Autodesk Inventor part; units mm, degrees
ref_plane "YZ Plane" through (0, 0, 0) normal (1, 0, 0) x (0, 1, 0)
ref_plane "XY Plane" through (0, 0, 0) normal (0, 0, 1) x (1, 0, 0)
sketch "Sketch1" plane through (0, 0, 0) normal (0, 0, 1) x (1, 0, 0)
  line L0 (0.9, 49.1) -> (0.9, 28.9)
  arc A0 (0.9, 49.1) -> (-0.9, 49.1) centre (0, 49.1) ccw
  line L1 (-0.9, 28.9) -> (-0.9, 49.1)
  arc A1 (-0.9, 28.9) -> (0.9, 28.9) centre (0, 28.9) ccw
  line L2 (0.9, 13.1) -> (0.9, -13.1)
  arc A2 (0.9, 13.1) -> (-0.9, 13.1) centre (0, 13.1) ccw
  line L3 (-0.9, -13.1) -> (-0.9, 13.1)
  arc A3 (-0.9, -13.1) -> (0.9, -13.1) centre (0, -13.1) ccw
  line L4 (0, 28.9) -> (0, 25.8465)
  arc A4 (0, 25.8465) -> (0.298, 23.4232) centre (10, 25.8465) ccw
  arc A5 (0.298, 18.5768) -> (0.298, 23.4232) centre (-9.4039, 21) ccw
  arc A6 (0.298, 18.5768) -> (0, 16.1535) centre (10, 16.1535) ccw
  line L5 (0, 16.1535) -> (0, 13.1)
  point P0 (0, 0)
  dimension "d0" = 10
  dimension "d1" = 10
ref_plane "Work Plane1" through (0, 28.9, 0) normal (0, 1, 0) x (-1, 0, 0)
sketch "Sketch2" plane through (0, 28.9, 0) normal (0, 1, 0) x (-1, 0, 0)
  line L0 (-0.5, 0) -> (0.5, 0)
  line L1 (0.5, 0) -> (0.5, -0.5)
  line L2 (0.5, -0.5) -> (-0.5, -0.5)
  line L3 (-0.5, -0.5) -> (-0.5, 0)
  point P0 (0, 0)
  point P1 (0, 0)
  dimension "d2" = 1
  dimension "d3" = 0.5
sweep "Sweep1" add profiles "Sketch2" path "Sketch1" path curves L4 A4 A5 A6 L5
properties part number "connector"
Verification items for the finished model (mm, model axes). Give positions to 0.01 mm unless a question says otherwise; leave off trailing zeros. Order: outer loops, then holes, each group sorted by start corner. A loop starts at its lowest first (then second) coordinate and runs counter-clockwise, first axis right, second up. Notation, with made-up numbers: M -22.5,-31.75 L 25.5,-31.75 A25 ccw 25.5,5.25 Z; hole C 6.25,42.5 d4. An arc over 180 degrees is marked long. Use one line per item in the form item = value. Start each with the question number.
Q1. Section check D-D (y = 23). Enter the section's corners in (x, z).
Q2. Section check C-C (y = 16.75). Enter the section's corners in (x, z), then the cut area to 3 significant figures.
Q3. Scan lines: line 1 along X through (y, z) = (15.75, -0.1); line 2 along X through (y, z) = (23.25, -0.1). Record each from-to range of solid material in increasing order. Write a range as [from, to].
Q4. Section check B-B (x = -0.05). Enter the section's corners in (y, z), then the cut area to 3 significant figures.
Q5. Section check A-A (z = -0.4). Enter the section's corners in (x, y), then the cut area to 3 significant figures.
Evaluation:
q1.outline = M -0.12,-0.5 L 0.9,-0.5 L 0.9,0 L -0.12,0 Z
q2.outline = M -0.48,-0.5 L 0.52,-0.5 L 0.52,0 L -0.48,0 Z
q2.area = 0.501 mm2
q3.line_1 = [-0.5, 0.5]
q3.line_2 = [-0.17, 0.85]
q4.outline = M 13.1,-0.5 L 19.34,-0.5 L 19.34,0 L 13.1,0 Z; M 22.66,-0.5 L 28.9,-0.5 L 28.9,0 L 22.66,0 Z
q4.area = 6.24 mm2
q5.outline = M -0.5,13.1 L 0.5,13.1 L 0.5,16.15 A9.5 cw 0.78,18.46 A10.5 ccw 0.78,23.54 A9.5 cw 0.5,25.85 L 0.5,28.9 L -0.5,28.9 L -0.5,25.85 A10.5 ccw -0.19,23.3 A9.5 cw -0.19,18.7 A10.5 ccw -0.5,16.15 Z
q5.area = 15.9 mm2
